Could you check a few things on this model? Use its own coordinates, in mm. Coordinates: 2 decimals unless noted, no trailing zeros. Write each loop counter-clockwise with the first axis right and the second up, starting at its lowest first coordinate (ties: lowest second). Pieces come first, ordered by that corner, then holes.
Item 1: I want a section at B-B on y = 6. Please give me the cut outline in (x, z).
Item 2: For P1, Ø2.5, axis at y = 12.5, z = 100, coming from the +X side; P2, Ø1, axis at y = 10, z = 164, coming from the -X side; P3, Ø10, axis at y = 14, z = 448.5, coming from the +X side, each with a flat end and sliding along its axis, tell me the tip position at first contact or that it passes through.
Item 3: I want a section at A-A on z = 437.5. Please give me the cut outline in (x, y).
Item 4: I want a section at C-C on x = 10. Please give me the cut outline in (y, z), then the cut area to 3 significant figures.
Item 5: If I drill on probe 1 along Y at (x, z) = (0.5, 400); probe 2 along Z at (x, y) = (0.8, 12.5); probe 3 along X at (y, z) = (6.5, 277.5), over which ranges is the centre line in solid material (lowest first)?
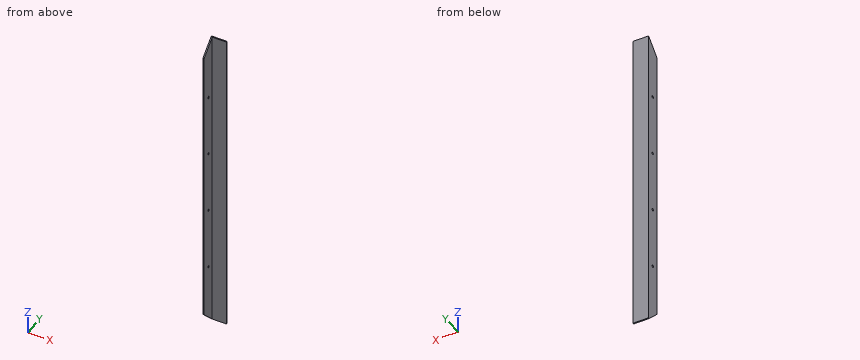
from build123d import *

# Parameters (mm, degrees)
BOSS_EXTRUDE1_DEPTH = 500
SKETCH2_R           = 2
CUT_EXTRUDE1_DEPTH  = 10
CUT_EXTRUDE2_DEPTH  = 10


with BuildPart() as part:
    # Sketch1 → Boss-Extrude1 (new body)
    with BuildSketch(Plane.XY):
        Polygon((0, 25), (0, 0), (2, 0), (2, 23), (25, 23), (25, 25), (5, 25), align=None)
    extrude(amount=BOSS_EXTRUDE1_DEPTH)

    # Sketch2 → Cut-Extrude1 (cut)
    with BuildSketch(Plane.ZY):
        with Locations(Location((100, 12.5, 0), (0, 0, 270))):
            Circle(SKETCH2_R)
        with Locations(Location((200, 12.5, 0), (0, 0, 270))):
            Circle(SKETCH2_R)
        with Locations(Location((300, 12.5, 0), (0, 0, 270))):
            Circle(SKETCH2_R)
        with Locations(Location((400, 12.5, 0), (0, 0, 270))):
            Circle(SKETCH2_R)
    extrude(amount=-CUT_EXTRUDE1_DEPTH, mode=Mode.SUBTRACT)

    # Sketch3 → Cut-Extrude2 (cut)
    with BuildSketch(Plane.ZY):
        Polygon((23, 0), (0, 23), (0, 0), align=None)
        Polygon((500, 23), (477, 0), (500, 0), align=None)
    extrude(amount=-CUT_EXTRUDE2_DEPTH, mode=Mode.SUBTRACT)


solid = part.part
Response values:
1. outline: (0, 17) - (2, 17) - (2, 483) - (0, 483) - close
2. P1: passes through
2. P2: stops at x = 0
2. P3: stops at x = 2
3. outline: (0, 0) - (2, 0) - (2, 23) - (25, 23) - (25, 25) - (0, 25) - close
4. outline: (23, 0) - (25, 0) - (25, 500) - (23, 500) - close
4. area: 1,000 mm2
5. probe 1: y = 0 to 10.5, 14.5 to 25
5. probe 2: z = 10.5 to 98, 102 to 198, 202 to 298, 302 to 398, 402 to 489.5
5. probe 3: x = 0 to 2
